Design review of the part built by this model. Coordinates are the model's own, in mm. A direction names the side the tool comes from. Give positions to 0.01 mm unless a question says otherwise; leave off trailing zeros. Loops run counter-clockwise (first coordinate to the right, second up) from the corner with the lowest first, then second, coordinate; pieces in that order, holes last. Notation, with made-up numbers: (84, 73) - (131, 73) arc R19 cw to (131, 83) - close; hole circle Ø8 at (-38, 23.25). An arc over 180 degrees is marked (long way). Write each question's results on one line, items separated by ' | '.
from build123d import *

# Parameters (mm, degrees)
F1_DEPTH = 16
F2_R     = 1
F3_R     = 1
F5_DEPTH = 1.5
F6_W     = 6
F6_H     = 16
F7_DEPTH = 1.5
F8_R     = 1.6
F9_DEPTH = 3


with BuildPart() as f1:
    # F0 (on Top) → F1 (new body)
    with BuildSketch(Plane.XY):
        Polygon((0, 1.5), (0, 45.5), (-1.5, 45.5), (-1.5, 0), (16, 0), (16, 1.5), align=None)
    extrude(amount=F1_DEPTH)

    # F2
    f2_edges = [f1.edges().sort_by_distance(p)[0] for p in [
        (-1.5, 0, 8),
    ]]
    fillet(f2_edges, radius=F2_R)

    # F3
    f3_edges = [f1.edges().sort_by_distance(p)[0] for p in [
        (0, 1.5, 8),
    ]]
    fillet(f3_edges, radius=F3_R)

    # F4 (on face) → F5 (cut)
    with BuildSketch(Plane(origin=(0, 1.5, 0), x_dir=(-1, 0, 0), z_dir=(0, 1, 0))):
        with BuildLine():
            ThreePointArc((-6.75, 5.6), (-8.35, 4), (-6.75, 2.4))
            Line((-6.75, 2.4), (-6.25, 2.4))
            ThreePointArc((-6.25, 2.4), (-4.65, 4), (-6.25, 5.6))
            Line((-6.25, 5.6), (-6.75, 5.6))
        make_face()
        with BuildLine():
            ThreePointArc((-6.75, 13.6), (-8.35, 12), (-6.75, 10.4))
            Line((-6.75, 10.4), (-6.25, 10.4))
            ThreePointArc((-6.25, 10.4), (-4.65, 12), (-6.25, 13.6))
            Line((-6.25, 13.6), (-6.75, 13.6))
        make_face()
    extrude(amount=-F5_DEPTH, mode=Mode.SUBTRACT)

    # F6 (on face) → F7 (join)
    with BuildSketch(Plane.YZ):
        with Locations((38.6, 8)):
            Rectangle(F6_W, F6_H)
        with Locations((18.6, 8)):
            Rectangle(F6_W, F6_H)
    extrude(amount=F7_DEPTH)

    # F8 (on face) → F9 (cut)
    with BuildSketch(Plane.YZ.offset(1.5)):
        with Locations((38.6, 12)):
            Circle(F8_R)
        with Locations((38.6, 4)):
            Circle(F8_R)
        with Locations((18.6, 12)):
            Circle(F8_R)
        with Locations((18.6, 4)):
            Circle(F8_R)
    extrude(amount=-F9_DEPTH, mode=Mode.SUBTRACT)


solid = f1.part
(1) Take a section at C-C on z = 1.5. Give the boundary of the cut face in (x, y).
Answers below:
outline: (-1.5, 1) arc R1 ccw to (-0.5, 0) - (16, 0) - (16, 1.5) - (1, 1.5) arc R1 cw to (0, 2.5) - (0, 15.6) - (1.5, 15.6) - (1.5, 21.6) - (0, 21.6) - (0, 35.6) - (1.5, 35.6) - (1.5, 41.6) - (0, 41.6) - (0, 45.5) - (-1.5, 45.5) - close
(2) Wall thickness on line 1 along Z through (x, y) = (-0.15, 38.6); line 2 along X through (y, z) = (21, 6.25); line 3 along Y through (x, z) = (14, 13.75): over which ranges is each line inside the solid? List them lowest first. Write a range as from..to.
Answers below:
line 1: 0..2.4, 5.6..10.4, 13.6..16 | line 2: -1.5..1.5 | line 3: 0..1.5
(3) Insertion check: P1, Ø1.8, axis at y = 19.5, z = 5.5, coming from the +X side; P2, Ø3, axis at x = 4, z = 5.5, coming from the +Y side; P3, Ø4.5, axis at y = 44.5, z = 11, coming from the +X side. Each pin has a flat end and moves straight along its axis. Give the tip position at first contact, or say it passes through.
Answers below:
P1: x = 1.5 | P2: y = 1.5 | P3: x = 0
(4) Take a section at A-A on y = 18.6. Give the boundary of the cut face in (x, z), plus the area to 3 significant figures.
Answers below:
outline: (-1.5, 0) - (1.5, 0) - (1.5, 2.4) - (-1.5, 2.4) - close; (-1.5, 5.6) - (1.5, 5.6) - (1.5, 10.4) - (-1.5, 10.4) - close; (-1.5, 13.6) - (1.5, 13.6) - (1.5, 16) - (-1.5, 16) - close | area: 28.8 mm2
(5) Take a section at D-D on x = 9.25. Give the boundary of the cut face in (y, z).
Answers below:
outline: (0, 0) - (1.5, 0) - (1.5, 16) - (0, 16) - close
(6) Take a section at B-B on z = 12. Give the boundary of the cut face in (x, y).
Answers below:
outline: (-1.5, 1) arc R1 ccw to (-0.5, 0) - (4.65, 0) - (4.65, 1.5) - (1, 1.5) arc R1 cw to (0, 2.5) - (0, 15.6) - (1.5, 15.6) - (1.5, 17) - (-1.5, 17) - close; (-1.5, 20.2) - (1.5, 20.2) - (1.5, 21.6) - (0, 21.6) - (0, 35.6) - (1.5, 35.6) - (1.5, 37) - (-1.5, 37) - close; (-1.5, 40.2) - (1.5, 40.2) - (1.5, 41.6) - (0, 41.6) - (0, 45.5) - (-1.5, 45.5) - close; (8.35, 0) - (16, 0) - (16, 1.5) - (8.35, 1.5) - close
(7) Tool access review of faces 5 (the cylindrical face through (4.65, 0.76, 11.96)), 6 (the flat face through (-1, 45.5, 8)), 7 (the flat face through (1, 15.6, 8)): name each direction out of +Z, -Z, +X, -X, +Y, -Y from which nothing blocks a thin tool from reaching the whole face with its end or side.
Answers below:
face 5: +Y, -Y | face 6: +Z, -Z, +X, -X, +Y | face 7: +Z, -Z, +X
(8) Draft analysis for pull direction X (two halves, no side actions). For faces 1 (the cylindrical face through (4.65, 0.76, 3.96)), 2 (the cylindrical face through (8.35, 0.76, 12.04)), 3 (the flat face through (8, 0, 8)), 4 (the flat face through (0, 9, 8)), state which applies: pulls with the +X half, pulls with the -X half, needs draft (parallel to the pull), parting line crosses it, or undercut.
Answers below:
face 1: undercut | face 2: undercut | face 3: needs draft | face 4: pulls with the +X half
